For this review, take the finished solid that the model builds, in its own axes (mm). Round coordinates to 2 decimals unless told otherwise and drop trailing zeros. Order: outer loops, then holes, each group sorted by start corner. A loop starts at its lowest first (then second) coordinate and runs counter-clockwise, first axis right, second up. Notation, with made-up numbers: (39.25, 55) - (47.25, 55) arc R23 cw to (47.25, 77) - close; hole circle Ø7 at (86, -5). An arc over 180 degrees is marked (long way). One line per item, written item: value.
```python
from build123d import *

# Parameters (mm, degrees)
SKETCH_281X300_10_R   = 1.6
SKETCH_281X300_10_R_2 = 15
SKETCH_281X300_10_R_3 = 2.15
SKETCH_281X300_10_R_4 = 2.2
F_4MM_DEPTH           = 4


with BuildPart() as part:
    # 底板轮廓_281x300_双槽内移10 → 凸台拉伸_4mm (new body)
    with BuildSketch(Plane.XY):
        with BuildLine():
            Line((-55.5, 83), (-55.5, 142))
            ThreePointArc((-55.5, 142), (-53.156854249, 147.656854249), (-47.5, 150))
            Line((-47.5, 150), (61.5, 150))
            ThreePointArc((61.5, 150), (67.156854249, 147.656854249), (69.5, 142))
            Line((69.5, 142), (69.5, 83))
            ThreePointArc((69.5, 83), (71.843145751, 77.343145751), (77.5, 75))
            Line((77.5, 75), (135.5, 75))
            ThreePointArc((135.5, 75), (139.035533906, 73.535533906), (140.5, 70))
            Line((140.5, 70), (140.5, -70))
            ThreePointArc((140.5, -70), (139.035533906, -73.535533906), (135.5, -75))
            Line((135.5, -75), (77.5, -75))
            ThreePointArc((77.5, -75), (71.843145751, -77.343145751), (69.5, -83))
            Line((69.5, -83), (69.5, -142))
            ThreePointArc((69.5, -142), (67.156854249, -147.656854249), (61.5, -150))
            Line((61.5, -150), (-47.5, -150))
            ThreePointArc((-47.5, -150), (-53.156854249, -147.656854249), (-55.5, -142))
            Line((-55.5, -142), (-55.5, -83))
            ThreePointArc((-55.5, -83), (-57.843145751, -77.343145751), (-63.5, -75))
            Line((-63.5, -75), (-138.5, -75))
            ThreePointArc((-138.5, -75), (-139.914213562, -74.414213562), (-140.5, -73))
            Line((-140.5, -73), (-140.5, -17))
            ThreePointArc((-140.5, -17), (-139.914213562, -15.585786438), (-138.5, -15))
            Line((-138.5, -15), (-132.5, -15))
            ThreePointArc((-132.5, -15), (-131.085786438, -14.414213562), (-130.5, -13))
            Line((-130.5, -13), (-130.5, 72))
            ThreePointArc((-130.5, 72), (-129.621320344, 74.121320344), (-127.5, 75))
            Line((-127.5, 75), (-63.5, 75))
            ThreePointArc((-63.5, 75), (-57.843145751, 77.343145751), (-55.5, 83))
        make_face()
        with Locations((100.5, -36)):
            Circle(SKETCH_281X300_10_R, mode=Mode.SUBTRACT)
        with Locations((130.5, -36)):
            Circle(SKETCH_281X300_10_R, mode=Mode.SUBTRACT)
        with Locations((100.5, 36)):
            Circle(SKETCH_281X300_10_R, mode=Mode.SUBTRACT)
        with Locations((7, 65.5)):
            Circle(SKETCH_281X300_10_R_2, mode=Mode.SUBTRACT)
        with Locations((7, 115)):
            Circle(SKETCH_281X300_10_R_3, mode=Mode.SUBTRACT)
        with Locations((-42.5, 65.5)):
            Circle(SKETCH_281X300_10_R_3, mode=Mode.SUBTRACT)
        with Locations((56.5, 65.5)):
            Circle(SKETCH_281X300_10_R_3, mode=Mode.SUBTRACT)
        with Locations((-40, 115)):
            Circle(SKETCH_281X300_10_R_3, mode=Mode.SUBTRACT)
        with Locations((130.5, 36)):
            Circle(SKETCH_281X300_10_R, mode=Mode.SUBTRACT)
        with Locations((49, 115)):
            Circle(SKETCH_281X300_10_R_3, mode=Mode.SUBTRACT)
        with Locations((7, 16)):
            Circle(SKETCH_281X300_10_R_3, mode=Mode.SUBTRACT)
        with Locations((31.290367902, -112.395183951)):
            Circle(SKETCH_281X300_10_R_4, mode=Mode.SUBTRACT)
        with Locations((-17.5, -112.395183951)):
            Circle(SKETCH_281X300_10_R_4, mode=Mode.SUBTRACT)
        with Locations((-17.5, -63.604816049)):
            Circle(SKETCH_281X300_10_R_4, mode=Mode.SUBTRACT)
        with Locations((31.290367902, -63.604816049)):
            Circle(SKETCH_281X300_10_R_4, mode=Mode.SUBTRACT)
        with Locations((7, 86.5)):
            Circle(SKETCH_281X300_10_R, mode=Mode.SUBTRACT)
        with Locations((25.186533479, 76)):
            Circle(SKETCH_281X300_10_R, mode=Mode.SUBTRACT)
        with Locations((100.5, -66)):
            Circle(SKETCH_281X300_10_R, mode=Mode.SUBTRACT)
        with Locations((25.186533479, 55)):
            Circle(SKETCH_281X300_10_R, mode=Mode.SUBTRACT)
        with Locations((100.5, 66)):
            Circle(SKETCH_281X300_10_R, mode=Mode.SUBTRACT)
        with Locations((7, 44.5)):
            Circle(SKETCH_281X300_10_R, mode=Mode.SUBTRACT)
        with Locations((130.5, 66)):
            Circle(SKETCH_281X300_10_R, mode=Mode.SUBTRACT)
        with Locations((130.5, -66)):
            Circle(SKETCH_281X300_10_R, mode=Mode.SUBTRACT)
        with Locations((-43, -105)):
            Circle(SKETCH_281X300_10_R, mode=Mode.SUBTRACT)
        with Locations((57, -57)):
            Circle(SKETCH_281X300_10_R, mode=Mode.SUBTRACT)
        with Locations((-43, -57)):
            Circle(SKETCH_281X300_10_R, mode=Mode.SUBTRACT)
        with Locations((57, -105)):
            Circle(SKETCH_281X300_10_R, mode=Mode.SUBTRACT)
        with Locations((-11.186533479, 55)):
            Circle(SKETCH_281X300_10_R, mode=Mode.SUBTRACT)
        with Locations((-11.186533479, 76)):
            Circle(SKETCH_281X300_10_R, mode=Mode.SUBTRACT)
        with Locations((130.5, 10)):
            Circle(SKETCH_281X300_10_R, mode=Mode.SUBTRACT)
        with Locations((130.5, -10)):
            Circle(SKETCH_281X300_10_R, mode=Mode.SUBTRACT)
        with Locations((-120.5, 10)):
            Circle(SKETCH_281X300_10_R, mode=Mode.SUBTRACT)
        with Locations((-120.5, -10)):
            Circle(SKETCH_281X300_10_R, mode=Mode.SUBTRACT)
        with Locations((-43, -115)):
            Circle(SKETCH_281X300_10_R, mode=Mode.SUBTRACT)
        with Locations((57, -67)):
            Circle(SKETCH_281X300_10_R, mode=Mode.SUBTRACT)
        with Locations((57, -115)):
            Circle(SKETCH_281X300_10_R, mode=Mode.SUBTRACT)
        with Locations((-43, -67)):
            Circle(SKETCH_281X300_10_R, mode=Mode.SUBTRACT)
        with Locations((-120.5, -66)):
            Circle(SKETCH_281X300_10_R, mode=Mode.SUBTRACT)
        with Locations((-90.5, -66)):
            Circle(SKETCH_281X300_10_R, mode=Mode.SUBTRACT)
        with Locations((-120.5, 66)):
            Circle(SKETCH_281X300_10_R, mode=Mode.SUBTRACT)
        with Locations((-90.5, 66)):
            Circle(SKETCH_281X300_10_R, mode=Mode.SUBTRACT)
        with Locations((-90.5, 36)):
            Circle(SKETCH_281X300_10_R, mode=Mode.SUBTRACT)
        with Locations((-120.5, 36)):
            Circle(SKETCH_281X300_10_R, mode=Mode.SUBTRACT)
        with Locations((-90.5, -36)):
            Circle(SKETCH_281X300_10_R, mode=Mode.SUBTRACT)
        with Locations((-120.5, -36)):
            Circle(SKETCH_281X300_10_R, mode=Mode.SUBTRACT)
        with BuildLine():
            Line((-25.5, -72), (-25.5, -104))
            ThreePointArc((-25.5, -104), (-24.914213562, -105.414213562), (-23.5, -106))
            Line((-23.5, -106), (42.5, -106))
            ThreePointArc((42.5, -106), (43.914213562, -105.414213562), (44.5, -104))
            Line((44.5, -104), (44.5, -72))
            ThreePointArc((44.5, -72), (43.914213562, -70.585786438), (42.5, -70))
            Line((42.5, -70), (-23.5, -70))
            ThreePointArc((-23.5, -70), (-24.914213562, -70.585786438), (-25.5, -72))
        make_face(mode=Mode.SUBTRACT)
        with BuildLine():
            Line((75.5, 50), (75.5, 36))
            ThreePointArc((75.5, 36), (80.5, 31), (85.5, 36))
            Line((85.5, 36), (85.5, 50))
            ThreePointArc((85.5, 50), (80.5, 55), (75.5, 50))
        make_face(mode=Mode.SUBTRACT)
        with BuildLine():
            Line((85.5, -50), (85.5, -36))
            ThreePointArc((85.5, -36), (80.5, -31), (75.5, -36))
            Line((75.5, -36), (75.5, -50))
            ThreePointArc((75.5, -50), (80.5, -55), (85.5, -50))
        make_face(mode=Mode.SUBTRACT)
        with BuildLine():
            Line((-95.5, -10), (-75.5, -10))
            ThreePointArc((-75.5, -10), (-65.5, 0), (-75.5, 10))
            Line((-75.5, 10), (-95.5, 10))
            ThreePointArc((-95.5, 10), (-105.5, 0), (-95.5, -10))
        make_face(mode=Mode.SUBTRACT)
    extrude(amount=F_4MM_DEPTH)


solid = part.part
```
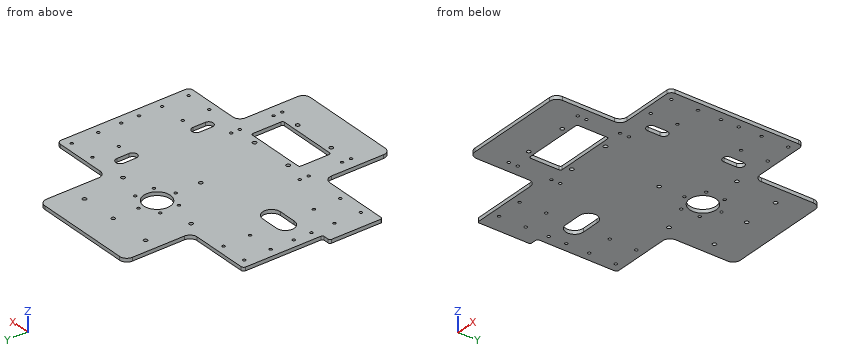
Item 1: Take a section at A-A (x = -81.5). Write out the cut boundary in (y, z), plus the area to 3 significant figures.
Returned:
outline: (-75, 0) - (-10, 0) - (-10, 4) - (-75, 4) - close; (10, 0) - (75, 0) - (75, 4) - (10, 4) - close
area: 520 mm^2
Item 2: Take a section at B-B (y = 60). Write out the cut boundary in (x, z).
Returned:
outline: (-130.5, 0) - (-6.96, 0) - (-6.96, 4) - (-130.5, 4) - close; (20.96, 0) - (140.5, 0) - (140.5, 4) - (20.96, 4) - close
Item 3: For P1, Ø2.5, axis at x = 57, y = -57, coming from the +Z side; P2, Ø5, axis at x = -42.5, y = 65.5, coming from the +Z side; P3, Ø2, axis at y = 32.5, z = 1, coming from the -X side, all flat-tipped, find the tip position at first contact; note any pin that passes through.
Returned:
P1: through
P2: z = 4
P3: x = -130.5
Item 4: Wall thickness on line 1 (Y direction, x = -43, z = 3); line 2 (Y direction, x = -90.5, z = 1.6); line 3 (X direction, y = -100, z = 1.15): over which ranges is each line inside the solid? List them lowest first.
Returned:
line 1: -150 to -116.6, -113.4 to -106.6, -103.4 to -68.6, -65.4 to -58.6, -55.4 to 63.41, 67.59 to 150
line 2: -75 to -67.6, -64.4 to -37.6, -34.4 to -10, 10 to 34.4, 37.6 to 64.4, 67.6 to 75
line 3: -55.5 to -25.5, 44.5 to 69.5
Item 5: Take a section at C-C (x = 95). Write out the cut boundary in (y, z).
Returned:
outline: (-75, 0) - (75, 0) - (75, 4) - (-75, 4) - close
Item 6: Take a section at D-D (z = 0.75). Count the separate pieces of the cut face and the enclosed holes in it, plus the area to 3 significant figures.
Returned:
separate pieces: 1
enclosed holes: 49
area: 55,200 mm^2
